Read the model definition and answer for the solid it produces. Units are mm, in the model's axes. Face numbers are marked on the shaded views. Round coordinates to 2 decimals unless told otherwise and drop trailing zeros. Order: outer loops, then holes, each group sorted by start corner. A loop starts at its lowest first (then second) coordinate and runs counter-clockwise, first axis right, second up. Notation, with made-up numbers: (76.5, 67.25) - (130.5, 67.25) arc R27 ccw to (130.5, 102.25) - close; hole circle Ø6 at (-35, 75). An arc over 180 degrees is marked (long way). Answer as a JSON object with one key per item and string values. Group by question number.
Q1. A cutting plane is placed at C-C on y = 36.5. Determine the outline of the cut face in (x, z), and give its area (3 significant figures).
Q2. Consider line 1 (Y direction, x = 10, z = 2); line 2 (X direction, y = 6.5, z = -0.5); line 3 (X direction, y = 23.5, z = 1). Determine where each line is inside the solid, lowest interval first.
Q3. Given pin 1 Ø5.5 at (x, z) = (0, 15) entering from +Y; pin 2 Ø8 at (x, z) = (12, -8.5) entering from -Y; pin 3 Ø4 at (y, z) = (15, -6) entering from -X; pin 4 Ø3 at (x, y) = (-9.5, 23.5) entering from -Z, each flat-ended and moving along its own axis, determine where each tip first touches the part or whether it passes through.
Q4. A cutting plane is placed at B-B on x = 15. Determine the outline of the cut face in (y, z).
Q5. The mould has two halves that part along X. Classify the marked faces 1, 2 and 3: pulls with the +X half, pulls with the -X half, needs draft (parallel to the pull), parting line crosses it, or undercut.
Q6. A cutting plane is placed at D-D on y = 15. Determine the outline of the cut face in (x, z).
Q7. A cutting plane is placed at A-A on z = 15. Determine the outline of the cut face in (x, y), and give its area (3 significant figures).
```python
from build123d import *

# Parameters (mm, degrees)
SKETCH1_R             = 10
BOSS_EXTRUDE1_DEPTH   = 40
SKETCH2_R             = 20
BOSS_EXTRUDE2_DEPTH   = 3
CIRPATTERN1_COUNT     = 4
M6_TAPPED_HOLE1_D     = 5
M6_TAPPED_HOLE1_DEPTH = 17
M6_TAPPED_HOLE1_TIP   = 1.502151548


with BuildPart() as part:
    # Sketch1 → Boss-Extrude1 (new body)
    with BuildSketch(Plane(origin=(0, 0, 0), x_dir=(1, 0, 0), z_dir=(0, 1, 0))):
        with Locations(Location((0, 0, 0), (0, 0, 270))):
            Circle(SKETCH1_R)
    extrude(amount=BOSS_EXTRUDE1_DEPTH)

    # Sketch2 → Boss-Extrude2 (add)
    with BuildSketch(Plane.XZ):
        with Locations(Location((0, 0, 0), (0, 0, 270))):
            Circle(SKETCH2_R)
    extrude(amount=-BOSS_EXTRUDE2_DEPTH)

    # Sketch3 → CSK for M3 Countersunk Flat Head Screw1 (revolve, cut)
    with BuildSketch(Plane(origin=(0, 3, -15), x_dir=(0, 0, 1), z_dir=(1, 0, 0))):
        Polygon((0, 0), (0, 3), (1.7, 3), (1.7, 1.45), (3.15, 0), align=None)
    csk_for_m3_countersunk_flat_head_screw1 = revolve(axis=Axis((0, 9.35, -15), (0, -1, 0)), mode=Mode.SUBTRACT)

    # CirPattern1: CSK for M3 Countersunk Flat Head Screw1 ×4 about axis
    cirpattern1_axis = Axis((0, 0, 0), (0, 1, 0))
    for i in range(1, CIRPATTERN1_COUNT):
        add(csk_for_m3_countersunk_flat_head_screw1.rotate(cirpattern1_axis, i * 360 / CIRPATTERN1_COUNT), mode=Mode.SUBTRACT)

    # M6 Tapped Hole1
    with Locations(Plane(origin=(0, 40, 0), x_dir=(1, 0, 0), z_dir=(0, 1, 0))):
        with Locations((0, 0)):
            Hole(M6_TAPPED_HOLE1_D / 2, depth=M6_TAPPED_HOLE1_DEPTH)
            with Locations((0, 0, -(M6_TAPPED_HOLE1_DEPTH + M6_TAPPED_HOLE1_TIP / 2))):  # 118° drill point
                Cone(0, M6_TAPPED_HOLE1_D / 2, M6_TAPPED_HOLE1_TIP, mode=Mode.SUBTRACT)


solid = part.part
```
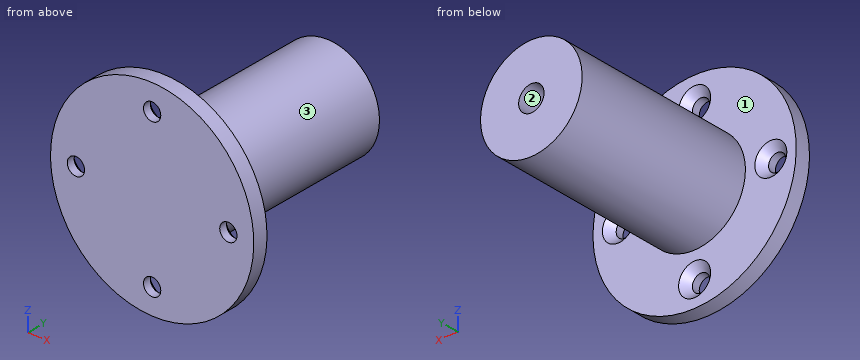
Result set:
{
 "1": {"outline": "circle Ø20 at (0, 0); hole circle Ø5 at (0, 0)", "area": "295 mm²"},
 "2": {"line 1": "y = 0 to 3", "line 2": "x = -9.99 to 9.99", "line 3": "x = -9.95 to -2.29, 2.29 to 9.95"},
 "3": {"pin 1": "stops at y = 2.6", "pin 2": "stops at y = 0", "pin 3": "stops at x = -9.17", "pin 4": "stops at z = -6"},
 "4": {"outline": "(0, -13.23) - (3, -13.23) - (3, -3.15) - (1.55, -1.7) - (0, -1.7) - close; (0, 1.7) - (1.55, 1.7) - (3, 3.15) - (3, 13.23) - (0, 13.23) - close"},
 "5": {"face 1": "needs draft", "face 2": "undercut", "face 3": "parting line crosses it"},
 "6": {"outline": "circle Ø20 at (0, 0)"},
 "7": {"outline": "(-13.23, 0) - (-1.7, 0) - (-1.7, 1.55) - (-3.15, 3) - (-13.23, 3) - close; (1.7, 0) - (13.23, 0) - (13.23, 3) - (3.15, 3) - (1.7, 1.55) - close", "area": "67.1 mm²"}
}
